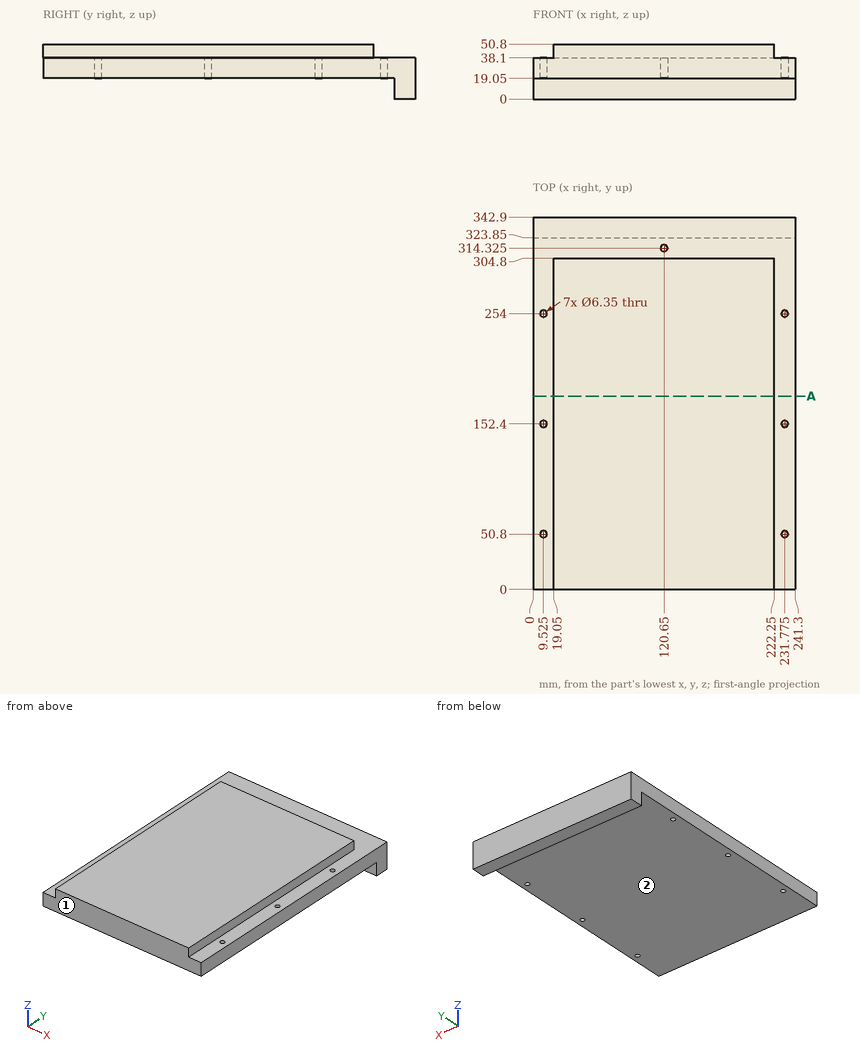
Source: three-view drawing plus pictorial views. Frame: mm from the lowest corner of the part. A direction names the side the tool comes from. Give positions to 0.01 mm unless a question says otherwise; leave off trailing zeros. Write each loop counter-clockwise with the first axis right and the second up, starting at its lowest first coordinate (ties: lowest second). Pieces come first, ordered by that corner, then holes. Notation, with made-up numbers: (-40, -12.5) -> (-33, -12.5) arc R23 ccw to (-33, 22.5) -> close; hole circle Ø10 at (-26, 31). An arc over 180 degrees is marked (long way). Write item = value, one per line.
Q1. Line query: line 1 (X direction, y = 254, z = 30); line 2 (Y direction, x = 120, z = 33); line 3 (X direction, y = 50, z = 33). Output: solid intervals per line, ascending. Write a range as from..to.
Here are the results:
line_1 = 0..6.35, 12.7..228.6, 234.95..241.3
line_2 = 0..311.22, 317.43..342.9
line_3 = 0..6.45, 12.6..228.7, 234.85..241.3
Q2. Reachability of the marked faces 1 and 2 from +Z, -Z, +X, -X, +Y, -Y: full face, straight path, thin tool, end or side. Return the list, or none.
Here are the results:
face_1 = +Z, -Z, +X, -X, -Y
face_2 = -Z, +X, -X, -Y
Q3. First-contact query: pin 1 (7.5 mm diameter, centred on x = 9.525, y = 152.4, fed in from +Z); pin 2 (8 mm diameter, centred on x = 164, y = 217.5, fed in from -Z); pin 3 (6 mm diameter, centred on x = 169.5, z = 9.5, fed in from -Y). Flat tips, straight axial feed; report the tip coordinate or a pass-through.
Here are the results:
pin_1 = 38.1
pin_2 = 19.05
pin_3 = 323.85
Q4. Cut plane A-A on y = 178. Return loops of the section in (x, z), then the cut area to 3 significant figures.
Here are the results:
outline = (0, 19.05) -> (241.3, 19.05) -> (241.3, 38.1) -> (222.25, 38.1) -> (222.25, 50.8) -> (19.05, 50.8) -> (19.05, 38.1) -> (0, 38.1) -> close
area = 7,180 mm²
